Autodesk Fusion 360 part; units mm, degrees
sketch "Sketch1" plane through (0, 0, 0) normal (0, 1, 0) x (1, 0, 0)
  line L0 (9.5, -7.75) -> (-9.5, -7.75)
  line L1 (-9.5, -7.75) -> (-9.5, 7.75)
  line L2 (-9.5, 7.75) -> (9.5, 7.75)
  line L3 (9.5, 7.75) -> (9.5, -7.75)
  line L4 (9.5, -7.75) -> (-9.5, 7.75) construction
  line L5 (-9.5, -7.75) -> (9.5, 7.75) construction
  dimension "d1" = 19
  dimension "d2" = 15.5
extrude "Extrude1" add sketch "Sketch1" along normal blind 15.5
fillet "Fillet1" radius 0.1 4 edges at (-9.5, 7.75, -7.75) (9.5, 7.75, -7.75) (9.5, 7.75, 7.75) (-9.5, 7.75, 7.75) 1 faces at (3.1667, 15.5, 2.5833)
sketch "Sketch2" plane through (0, 0, 0) normal (0, -1, 0) x (1, 0, 0)
  arc A0 (9.5, 7.65) -> (9.4, 7.75) centre (9.4, 7.65) ccw
  line L0 (9.4, 7.75) -> (-9.4, 7.75)
  arc A1 (-9.4, 7.75) -> (-9.5, 7.65) centre (-9.4, 7.65) ccw
  line L1 (-9.5, 7.65) -> (-9.5, -7.65)
  arc A2 (-9.5, -7.65) -> (-9.4, -7.75) centre (-9.4, -7.65) ccw
  line L2 (-9.4, -7.75) -> (9.4, -7.75)
  arc A3 (9.4, -7.75) -> (9.5, -7.65) centre (9.4, -7.65) ccw
  line L3 (9.5, -7.65) -> (9.5, 7.65)
  line L4 (6.1, 6) -> (-6.1, 6) construction
  line L5 (-6.1, 6) -> (-6.1, -6) construction
  line L6 (-6.1, -6) -> (6.1, -6) construction
  line L7 (6.1, -6) -> (6.1, 6) construction
  line L8 (6.1, 6) -> (-6.1, -6) construction
  line L9 (-6.1, 6) -> (6.1, -6) construction
  line L10 (-6.1, 0) -> (-8.1, 0) construction
  line L11 (-5.6, 5.75) -> (-6.6, 5.75)
  line L12 (-6.6, 5.75) -> (-6.6, 6.25)
  line L13 (-6.6, 6.25) -> (-5.6, 6.25)
  line L14 (-5.6, 6.25) -> (-5.6, 5.75)
  line L15 (-5.6, 5.75) -> (-6.6, 6.25) construction
  line L16 (-6.6, 5.75) -> (-5.6, 6.25) construction
  line L17 (-5.6, -5.75) -> (-6.6, -5.75)
  line L18 (-6.6, -5.75) -> (-6.6, -6.25)
  line L19 (-6.6, -6.25) -> (-5.6, -6.25)
  line L20 (-5.6, -6.25) -> (-5.6, -5.75)
  line L21 (-5.6, -5.75) -> (-6.6, -6.25) construction
  line L22 (-6.6, -5.75) -> (-5.6, -6.25) construction
  line L23 (6.6, 6.25) -> (5.6, 6.25)
  line L24 (5.6, 6.25) -> (5.6, 5.75)
  line L25 (5.6, 5.75) -> (6.6, 5.75)
  line L26 (6.6, 5.75) -> (6.6, 6.25)
  line L27 (6.6, 6.25) -> (5.6, 5.75) construction
  line L28 (5.6, 6.25) -> (6.6, 5.75) construction
  line L29 (6.6, -5.75) -> (5.6, -5.75)
  line L30 (5.6, -5.75) -> (5.6, -6.25)
  line L31 (5.6, -6.25) -> (6.6, -6.25)
  line L32 (6.6, -6.25) -> (6.6, -5.75)
  line L33 (6.6, -5.75) -> (5.6, -6.25) construction
  line L34 (5.6, -5.75) -> (6.6, -6.25) construction
  line L35 (-7.85, -0.5) -> (-8.35, -0.5)
  line L36 (-8.35, -0.5) -> (-8.35, 0.5)
  line L37 (-8.35, 0.5) -> (-7.85, 0.5)
  line L38 (-7.85, 0.5) -> (-7.85, -0.5)
  line L39 (-7.85, -0.5) -> (-8.35, 0.5) construction
  line L40 (-8.35, -0.5) -> (-7.85, 0.5) construction
  point P0 (-6.1, 6)
  point P1 (-6.1, -6)
  point P2 (6.1, 6)
  point P3 (6.1, -6)
  point P4 (-8.1, 0)
  dimension "d7" = 12.2
  dimension "d8" = 12
  dimension "d9" = 2
  dimension "d10" = 1
  dimension "d11" = 0.5
  dimension "d12" = 1
  dimension "d13" = 0.5
  dimension "d14" = 1
  dimension "d15" = 0.5
  dimension "d16" = 1
  dimension "d17" = 0.5
  dimension "d18" = 0.5
  dimension "d19" = 1
extrude "Extrude2" add sketch "Sketch2" along normal blind 4.5 contours L11 L12 L13 L14 | L17 L18 L19 L20 | L23 L24 L25 L26 | L29 L30 L31 L32 | L35 L36 L37 L38
sketch "Sketch3" plane through (0, 0, 0) normal (0, -1, 0) x (1, 0, 0)
  line L0 (6.6, -6.25) -> (5.6, -6.25)
  line L1 (5.6, -6.25) -> (5.6, -5.75)
  line L2 (5.6, -5.75) -> (6.6, -5.75)
  line L3 (6.6, -5.75) -> (6.6, -6.25)
  line L4 (-5.6, -6.25) -> (-6.6, -6.25)
  line L5 (-6.6, -6.25) -> (-6.6, -5.75)
  line L6 (-6.6, -5.75) -> (-5.6, -5.75)
  line L7 (-5.6, -5.75) -> (-5.6, -6.25)
  line L8 (6.6, 5.75) -> (5.6, 5.75)
  line L9 (5.6, 5.75) -> (5.6, 6.25)
  line L10 (5.6, 6.25) -> (6.6, 6.25)
  line L11 (6.6, 6.25) -> (6.6, 5.75)
  line L12 (-7.85, 0.5) -> (-7.85, -0.5)
  line L13 (-7.85, -0.5) -> (-8.35, -0.5)
  line L14 (-8.35, -0.5) -> (-8.35, 0.5)
  line L15 (-8.35, 0.5) -> (-7.85, 0.5)
  line L16 (-5.6, 6.25) -> (-5.6, 5.75)
  line L17 (-5.6, 5.75) -> (-6.6, 5.75)
  line L18 (-6.6, 5.75) -> (-6.6, 6.25)
  line L19 (-6.6, 6.25) -> (-5.6, 6.25)
  arc A0 (9.5, 7.65) -> (9.4, 7.75) centre (9.4, 7.65) ccw
  line L20 (9.4, 7.75) -> (-9.4, 7.75)
  arc A1 (-9.4, 7.75) -> (-9.5, 7.65) centre (-9.4, 7.65) ccw
  line L21 (-9.5, 7.65) -> (-9.5, -7.65)
  arc A2 (-9.5, -7.65) -> (-9.4, -7.75) centre (-9.4, -7.65) ccw
  line L22 (-9.4, -7.75) -> (9.4, -7.75)
  arc A3 (9.4, -7.75) -> (9.5, -7.65) centre (9.4, -7.65) ccw
  line L23 (9.5, -7.65) -> (9.5, 7.65)
  circle A4 centre (-6.5, 0) radius 0.65
  dimension "d22" = 1.3
extrude "Extrude3" cut sketch "Sketch3" against normal blind 0.1 contours A4
sketch "Sketch4" plane through (0, 0.1, 0) normal (0, -1, 0) x (1, 0, 0)
  circle A0 centre (-6.5, 0) radius 0.65
  circle A1 centre (-6.5, 0) radius 0.15
  dimension "d25" = 0.3
extrude "Extrude4" add sketch "Sketch4" along normal blind 0.1 contours A1
sketch "Sketch5" plane through (0, 15.5, 0) normal (0, 1, 0) x (-1, 0, 0)
  line L0 (9.4, 7.65) -> (-9.4, 7.65)
  line L1 (-9.4, 7.65) -> (-9.4, -7.65)
  line L2 (-9.4, -7.65) -> (9.4, -7.65)
  line L3 (9.4, -7.65) -> (9.4, 7.65)
  line L4 (10.1, 1.25) -> (8.7, 1.25)
  line L5 (8.7, 1.25) -> (8.7, -1.25)
  line L6 (8.7, -1.25) -> (10.1, -1.25)
  line L7 (10.1, -1.25) -> (10.1, 1.25)
  line L8 (10.1, 1.25) -> (8.7, -1.25) construction
  line L9 (8.7, 1.25) -> (10.1, -1.25) construction
  point P0 (9.4, 0)
  dimension "d28" = 1.4
  dimension "d29" = 2.5
extrude "Extrude5" cut sketch "Sketch5" against normal blind 0.2 contours L3 L4 L6 L7 | L3 L4 L5 L6
sketch "Sketch6" plane through (0, 15.5, 0) normal (0, 1, 0) x (-1, 0, 0)
  line L0 (8.7, 1.25) -> (9.4, 1.25)
  line L1 (9.4, 1.25) -> (9.4, 7.65)
  line L2 (9.4, 7.65) -> (-9.4, 7.65)
  line L3 (-9.4, 7.65) -> (-9.4, -7.65)
  line L4 (-9.4, -7.65) -> (9.4, -7.65)
  line L5 (9.4, -7.65) -> (9.4, -1.25)
  line L6 (9.4, -1.25) -> (8.7, -1.25)
  line L7 (8.7, -1.25) -> (8.7, 1.25)
  circle A0 centre (8.725, 6.9131) radius 0.5
  dimension "d32" = 1
extrude "Extrude6" cut sketch "Sketch6" against normal blind 0.2 contours A0
Could you check a few things on this model? Use its own coordinates, in mm. A direction names the side the tool comes from. Give positions to 0.01 mm unless a question says otherwise; leave off trailing zeros. Loops run counter-clockwise (first coordinate to the right, second up) from the corner with the lowest first, then second, coordinate; pieces in that order, holes last. Notation, with made-up numbers: (44, 17) -> (84, 17) arc R38 ccw to (84, 56) -> close; hole circle Ø11 at (41.5, -31.5). An arc over 180 degrees is marked (long way). Put each result on its own line as item: value.
(1) Please list where this line runs through material, in increasing order: probe 1 along Y at (x, z) = (-3.25, -1.75). Write a range as [from, to].
Computed:
probe 1: [0, 15.5]
(2) For faces 1 (the face through (6, -2, -6.25)), 2 (the face through (-6, -2, -5.75)), 3 (the face through (-9, 15.3, 0)), 4 (the face through (-9, 15.3, 7)), which set-ups out of +Z, -Z, +X, -X, +Y, -Y let a thin tool reach every point of the face, with its end or its side?
Computed:
face 1: -Z, +X, -X, -Y
face 2: +X, -X, -Y
face 3: -X, +Y
face 4: +Y
(3) I'm going to push flat-ended pins straight in: pin 1 Ø1.1 at (x, y) = (-6, -2.5) entering from -Z; pin 2 Ø4.5 at (x, z) = (-3.5, -2) entering from -Y; pin 3 Ø0.8 at (x, y) = (6, -1.5) entering from +Z. Where does each tip first touch, or does it pass through?
Computed:
pin 1: z = -6.25
pin 2: y = 0
pin 3: z = 6.25
(4) Thinking about a two-plate mould opening in Z: for faces 5 (the face through (0, 8, -7.75)), 6 (the face through (-6, -2, 5.75)), 7 (the face through (-7, 0.1, 0)), 8 (the face through (-7.85, -2, 0)), which applies, pulls with the +Z half, pulls with the -Z half, needs draft (parallel to the pull), parting line crosses it, or undercut?
Computed:
face 5: pulls with the -Z half
face 6: undercut
face 7: undercut
face 8: needs draft
(5) Imagine slicing it at A-A on x = 1. Write out the boundary of the cut face in (y, z).
Computed:
outline: (0, -7.75) -> (15.4, -7.75) arc R0.1 ccw to (15.5, -7.65) -> (15.5, 7.65) arc R0.1 ccw to (15.4, 7.75) -> (0, 7.75) -> close
